from build123d import *

# Parameters (mm, degrees)
F1_DEPTH = 6.35


with BuildPart() as f1:
    # F0 (on Top) → F1 (new body)
    with BuildSketch(Plane.XY):
        with BuildLine():
            ThreePointArc((9.525, 0), (6.7351920908, 6.7351920908), (0, 9.525))
            ThreePointArc((0, 9.525), (-6.7351920908, 6.7351920908), (-9.525, 0))
            ThreePointArc((-9.525, 0), (0, -9.525), (9.525, 0))
        make_face()
        with BuildLine():
            ThreePointArc((3.175, 0), (-2.2450640303, -2.2450640303), (0, 3.175))
            ThreePointArc((0, 3.175), (2.2450640303, 2.2450640303), (3.175, 0))
        make_face(mode=Mode.SUBTRACT)
        with BuildLine():
            ThreePointArc((-9.525, 0), (-6.7351920908, 6.7351920908), (0, 9.525))
            Line((0, 9.525), (0, 17.430102046))
            ThreePointArc((0, 17.430102046), (-6.7351920908, 20.2199099552), (-9.525, 26.955102046))
            Line((-9.525, 26.955102046), (-9.525, 0))
        make_face()
        with BuildLine():
            Line((0, 17.430102046), (0, 9.525))
            ThreePointArc((0, 9.525), (6.7351920908, 6.7351920908), (9.525, 0))
            Line((9.525, 0), (9.525, 26.955102046))
            ThreePointArc((9.525, 26.955102046), (6.7351920908, 20.2199099552), (0, 17.430102046))
        make_face()
        with BuildLine():
            ThreePointArc((-9.525, 26.955102046), (-6.7351920908, 20.2199099552), (0, 17.430102046))
            Line((0, 17.430102046), (0, 23.780102046))
            ThreePointArc((0, 23.780102046), (-2.2450640303, 29.2001660763), (3.175, 26.955102046))
            Line((3.175, 26.955102046), (9.525, 26.955102046))
            ThreePointArc((9.525, 26.955102046), (0, 36.480102046), (-9.525, 26.955102046))
        make_face()
        with BuildLine():
            Line((0, 23.780102046), (0, 17.430102046))
            ThreePointArc((0, 17.430102046), (6.7351920908, 20.2199099552), (9.525, 26.955102046))
            Line((9.525, 26.955102046), (3.175, 26.955102046))
            ThreePointArc((3.175, 26.955102046), (2.2450640303, 24.7100380157), (0, 23.780102046))
        make_face()
    extrude(amount=F1_DEPTH)


solid = f1.part
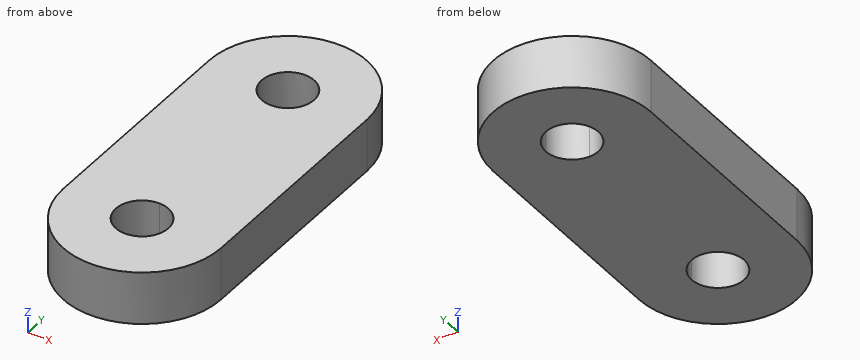
The listing builds one solid part. Answer for the finished solid, in the listing's coordinates (mm). Coordinates: 2 decimals unless noted, no trailing zeros. Write each loop counter-clockwise with the first axis right and the second up, starting at its lowest first coordinate (ties: lowest second). Pieces come first, ordered by that corner, then holes. Notation, with made-up numbers: M 78,-40 L 124,-40 A24 cw 124,-23 Z; hole C 14.5,65 d4. An arc over 180 degrees is marked long. Put each result on its own line as item: value. Start each with the question number.
1. Consider line 1 (Y direction, x = 0, z = 4.25) (3 decimals); line 2 (Y direction, x = -2.75, z = 3.5); line 3 (X direction, y = -2.5, z = 5.25). Determine where each line is inside the solid, lowest interval first. Write a range as from..to.
2. A cutting plane is placed at A-A on z = 2. Write down the section's boundary in (x, y) (3 decimals).
3. A cutting plane is placed at B-B on x = -2.25. Write down the section's boundary in (y, z), then the cut area to 3 significant figures.
4. A cutting plane is placed at C-C on y = 26. Write down the section's boundary in (x, z) (3 decimals), then the cut area to 3 significant figures.
5. A cutting plane is placed at D-D on x = -7.5. Write down the section's boundary in (y, z), then the cut area to 3 significant figures.
6. Flat-ended cylindrical pins translate along their axes: P1, Ø1.5, axis at x = -2.5, z = 5, coming from the -Y side; P2, Ø1.5, axis at x = 3.5, z = 4.5, coming from the +Y side; P3, Ø2, axis at x = 7, z = 3, coming from the +Y side; P4, Ø10, axis at x = 0, y = 0, coming from the +Z side. Find the tip coordinate at first contact, or state that the pin passes through.
Resolved:
1. line 1: y = -9.525..-3.175, 3.175..23.78, 30.13..36.48
1. line 2: y = -9.12..-1.59, 1.59..25.37, 28.54..36.07
1. line 3: x = -9.19..-1.96, 1.96..9.19
2. outline: M -9.525,0 A9.525 ccw 9.525,0 L 9.525,26.955 A9.525 ccw -9.525,26.955 Z; hole C 0,0 d6.35; hole C 0,26.955 d6.35
3. outline: M -9.26,0 L -2.24,0 L -2.24,6.35 L -9.26,6.35 Z; M 2.24,0 L 24.71,0 L 24.71,6.35 L 2.24,6.35 Z; M 29.2,0 L 36.21,0 L 36.21,6.35 L 29.2,6.35 Z
3. area: 232 mm2
4. outline: M -9.525,0 L -3.028,0 L -3.028,6.35 L -9.525,6.35 Z; M 3.028,0 L 9.525,0 L 9.525,6.35 L 3.028,6.35 Z
4. area: 82.5 mm2
5. outline: M -5.87,0 L 32.83,0 L 32.83,6.35 L -5.87,6.35 Z
5. area: 246 mm2
6. P1: stops at y = -9.36
6. P2: stops at y = 36.07
6. P3: stops at y = 34.35
6. P4: stops at z = 6.35
